Verification items for the finished model (mm, model axes). A direction names the side the tool comes from. Coordinates: 2 decimals unless noted, no trailing zeros. Order: outer loops, then holes, each group sorted by start corner. A loop starts at its lowest first (then second) coordinate and runs counter-clockwise, first axis right, second up. Notation, with made-up numbers: (-30.75, 18) - (-24.75, 18) arc R12 cw to (-24.75, 34) - close; hole circle Ø1 at (-24.75, 23.5). An arc over 180 degrees is marked (long way). Answer as CSV lines item,"result". Start each with the question number.
1. Mould release check, pull along X, two halves, no side actions. Record for faces 3 (the flat face through (20.69, -39, 5)), 4 (the flat face through (-38.3, 5.6, 0)), 5 (the cylindrical face through (-40.9, -36.63, 4.51)): pulls with the +X half, pulls with the -X half, needs draft (parallel to the pull), parting line crosses it, or undercut.
2. Material ranges on L1, parallel to Y at x = 25, z = 3.25; L2, parallel to X at y = -31.5, z = 0.75; L3, parallel to Y at x = -44, z = 5.75, recorded low to high. Write a range as [from, to].
3. Section check D-D (y = 45). Record the cut outline in (x, z), and give its area (3 significant figures).
4. Section check C-C (z = 4.75). Count the separate pieces of the cut face and the enclosed holes in it, and give its area (3 significant figures).
5. Section check A-A (y = 3). Record the cut outline in (x, z), and give its area (3 significant figures).
6. Set-up check for faces 1 (the flat face through (26, -47.479, 5)), 2 (the flat face through (-37.9, -1, 5)): record each of +Z, -Z, +X, -X, +Y, -Y from which the full face is reachable in a straight line by a thin tool's end or side.
7. Go/stop test with flat-tipped pins: pin 1 (3 mm diameter, centred on x = 26.5, z = 7.5, fed in from +Y); pin 2 (2 mm diameter, centred on y = 0.5, z = 4.5, fed in from +X); pin 3 (1.2 mm diameter, centred on y = -41.5, z = 5, fed in from +X). Record where each tip stops, or that it passes through.
8. Section check B-B (x = 0). Record the cut outline in (y, z), and give its area (3 significant figures).
from build123d import *

# Parameters (mm, degrees)
F1_DEPTH = 9.144


with BuildPart() as f1:
    # F0 (on Top) → F1 (new body)
    with BuildSketch(Plane.XY):
        with BuildLine():
            Line((26.232975, -53.528168), (34.841218, -44.634543))
            ThreePointArc((34.841218, -44.634543), (36.919466, -41.859873), (37.011544, -38.394412))
            Line((37.011544, -38.394412), (37.011544, -23.138775))
            Line((37.011544, -23.138775), (37.011544, 46.751468))
            Line((37.011544, 46.751468), (8.889462, 47.060993))
            ThreePointArc((8.889462, 47.060993), (0.097842, 56.048297), (-8.889462, 47.256677))
            Line((-8.889462, 47.256677), (-43.862213, 47.641603))
            Line((-43.862213, 47.641603), (-43.862213, -30.166319))
            ThreePointArc((-43.862213, -30.166319), (-60.287374, -46.719226), (-37.899839, -40.193666))
            Line((-37.899839, -40.193666), (-37.899839, 40.192322))
            Line((-37.899839, 40.192322), (31.105572, 40.192322))
            Line((31.105572, 40.192322), (30.562247, -34.348597))
            ThreePointArc((30.562247, -34.348597), (27.948657, -35.522102), (26.232975, -37.816531))
            ThreePointArc((26.232975, -37.816531), (17.395999, -35.502474), (17.624733, -44.634543))
            Line((17.624733, -44.634543), (26.232975, -53.528168))
        make_face()
        with BuildLine():
            Line((-52.031719, -43.74671), (-52.031719, -50.194425))
            ThreePointArc((-52.031719, -50.194425), (-54.56503, -49.26521), (-56.75136, -47.683736))
            Line((-56.75136, -47.683736), (-52.031719, -43.74671))
        make_face(mode=Mode.SUBTRACT)
        with BuildLine():
            ThreePointArc((-43.121746, -47.683736), (-45.308076, -49.26521), (-47.841386, -50.194425))
            Line((-47.841386, -50.194425), (-47.841386, -43.74671))
            Line((-47.841386, -43.74671), (-43.121746, -47.683736))
        make_face(mode=Mode.SUBTRACT)
        with BuildLine():
            Line((-52.031719, -30.934597), (-52.031719, -40.564511))
            Line((-52.031719, -40.564511), (-58.280842, -45.808346))
            ThreePointArc((-58.280842, -45.808346), (-59.022402, -36.747142), (-52.031719, -30.934597))
        make_face(mode=Mode.SUBTRACT)
        with BuildLine():
            Line((-41.59198, -45.807894), (-47.841386, -40.564511))
            Line((-47.841386, -40.564511), (-47.841386, -30.934597))
            ThreePointArc((-47.841386, -30.934597), (-40.850807, -36.746896), (-41.59198, -45.807894))
        make_face(mode=Mode.SUBTRACT)
        with BuildLine():
            Line((18.88916, -42.058198), (20.690326, -40.490497))
            Line((20.690326, -40.490497), (20.690326, -42.892432))
            ThreePointArc((20.690326, -42.892432), (19.716707, -42.633005), (18.88916, -42.058198))
        make_face(mode=Mode.SUBTRACT)
        with BuildLine():
            Line((21.198326, -42.892432), (21.198326, -40.490497))
            Line((21.198326, -40.490497), (23.02938, -42.028172))
            ThreePointArc((23.02938, -42.028172), (22.191134, -42.624032), (21.198326, -42.892432))
        make_face(mode=Mode.SUBTRACT)
        with BuildLine():
            Line((22.422975, -47.479119), (26.232975, -47.479119))
            Line((26.232975, -47.479119), (30.042975, -47.479119))
            ThreePointArc((30.042975, -47.479119), (26.232975, -50.106314), (22.422975, -47.479119))
        make_face(mode=Mode.SUBTRACT)
        with BuildLine():
            Line((29.510517, -42.100913), (31.267625, -40.490497))
            Line((31.267625, -40.490497), (31.267625, -42.892432))
            ThreePointArc((31.267625, -42.892432), (30.321915, -42.645753), (29.510517, -42.100913))
        make_face(mode=Mode.SUBTRACT)
        with BuildLine():
            ThreePointArc((33.532733, -42.100913), (32.721335, -42.645753), (31.775625, -42.892432))
            Line((31.775625, -42.892432), (31.775625, -40.490497))
            Line((31.775625, -40.490497), (33.532733, -42.100913))
        make_face(mode=Mode.SUBTRACT)
        with BuildLine():
            ThreePointArc((18.605909, -41.732939), (18.277879, -38.789893), (20.690326, -37.072561))
            Line((20.690326, -37.072561), (20.690326, -39.982497))
            Line((20.690326, -39.982497), (18.605909, -41.732939))
        make_face(mode=Mode.SUBTRACT)
        with BuildLine():
            ThreePointArc((21.198326, -37.072561), (23.610772, -38.789893), (23.282742, -41.732939))
            Line((23.282742, -41.732939), (21.198326, -39.982497))
            Line((21.198326, -39.982497), (21.198326, -37.072561))
        make_face(mode=Mode.SUBTRACT)
        with BuildLine():
            ThreePointArc((29.255999, -41.826183), (28.831577, -38.844128), (31.267625, -37.072561))
            Line((31.267625, -37.072561), (31.267625, -39.982497))
            Line((31.267625, -39.982497), (29.255999, -41.826183))
        make_face(mode=Mode.SUBTRACT)
        with BuildLine():
            Line((31.775625, -39.982497), (31.775625, -37.072561))
            ThreePointArc((31.775625, -37.072561), (34.211673, -38.844128), (33.787252, -41.826183))
            Line((33.787252, -41.826183), (31.775625, -39.982497))
        make_face(mode=Mode.SUBTRACT)
        with BuildLine():
            ThreePointArc((-5.714654, 47.221733), (0.062898, 52.873489), (5.714654, 47.095937))
            Line((5.714654, 47.095937), (-5.714654, 47.221733))
        make_face(mode=Mode.SUBTRACT)
    extrude(amount=F1_DEPTH)


solid = f1.part
Evaluation:
1,face 3,"undercut"
1,face 4,"needs draft"
1,face 5,"undercut"
2,L1,"y = [-52.25, -49.92], [-47.48, -35.96], [40.19, 46.88]"
2,L2,"x = [-57.86, -53.8], [-52.03, -47.84], [-46.07, -37.9], [30.58, 37.01]"
2,L3,"y = [-51.04, -48.43], [-46.95, -43.79], [-32.7, -30.09]"
3,outline,"(-43.86, 0) - (37.01, 0) - (37.01, 9.14) - (-43.86, 9.14) - close"
3,area,"740 mm²"
4,separate pieces,"1"
4,enclosed holes,"14"
4,area,"2,030 mm²"
5,outline,"(-43.86, 0) - (-37.9, 0) - (-37.9, 9.14) - (-43.86, 9.14) - close; (30.83, 0) - (37.01, 0) - (37.01, 9.14) - (30.83, 9.14) - close"
5,area,"111 mm²"
6,face 1,"+Z, -Z"
6,face 2,"+Z, -Z, -Y"
7,pin 1,"stops at y = 46.88"
7,pin 2,"stops at x = 37.01"
7,pin 3,"stops at x = 37.16"
8,outline,"(40.19, 0) - (47.16, 0) - (47.16, 9.14) - (40.19, 9.14) - close; (52.87, 0) - (56.05, 0) - (56.05, 9.14) - (52.87, 9.14) - close"
8,area,"92.7 mm²"
